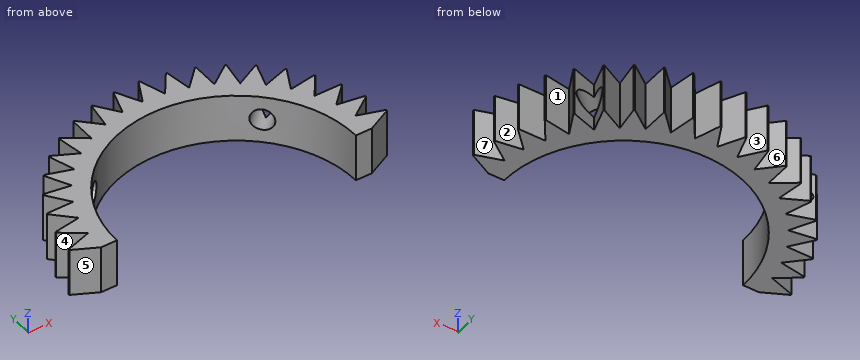
from build123d import *

# Parameters (mm, degrees)
BOSS_EXTRUDE1_DEPTH    = 7.5
CUT_EXTRUDE1_DEPTH     = 7.5
M8X1_25_TAPPED_HOLE4_D = 6.8
M8X1_25_TAPPED_HOLE5_D = 6.8


with BuildPart() as part:
    # Sketch1 → Boss-Extrude1 (new body, symmetric)
    with BuildSketch(Plane.XY):
        with BuildLine():
            Line((-50, 0), (-37.5, 0))
            ThreePointArc((-37.5, 0), (0, 37.5), (37.5, 0))
            Line((37.5, 0), (50, 0))
            ThreePointArc((50, 0), (0, 50), (-50, 0))
        make_face()
    extrude(amount=BOSS_EXTRUDE1_DEPTH, both=True)

    # Sketch2 → Cut-Extrude1 (cut, symmetric)
    with BuildSketch(Plane.XY):
        with BuildLine():
            Line((-3.75, 49.859176688), (0, 42.5))
            Line((0, 42.5), (3.75, 49.859176688))
            ThreePointArc((3.75, 49.859176688), (0, 50), (-3.75, 49.859176688))
        make_face()
        with BuildLine():
            Line((4.095862355, 49.83195673), (6.648464764, 41.976754475))
            Line((6.648464764, 41.976754475), (11.50352491, 48.658698242))
            ThreePointArc((11.50352491, 48.658698242), (7.821723252, 49.38441703), (4.095862355, 49.83195673))
        make_face()
        with BuildLine():
            Line((11.840870986, 48.577708615), (13.133222261, 40.419901943))
            Line((13.133222261, 40.419901943), (18.973794858, 46.260081157))
            ThreePointArc((18.973794858, 46.260081157), (15.450849719, 47.552825815), (11.840870986, 48.577708615))
        make_face()
        with BuildLine():
            Line((19.294318075, 46.127316094), (19.294596239, 37.867777278))
            Line((19.294596239, 37.867777278), (25.976867007, 42.722387346))
            ThreePointArc((25.976867007, 42.722387346), (22.699524987, 44.550326209), (19.294318075, 46.127316094))
        make_face()
        with BuildLine():
            Line((26.27267502, 42.541115962), (24.980873222, 34.383222261))
            Line((24.980873222, 34.383222261), (32.340302478, 38.13272657))
            ThreePointArc((32.340302478, 38.13272657), (29.389262615, 40.450849719), (26.27267502, 42.541115962))
        make_face()
        with BuildLine():
            Line((32.604111511, 37.90741237), (30.0520382, 30.0520382))
            Line((30.0520382, 30.0520382), (37.90741237, 32.604111511))
            ThreePointArc((37.90741237, 32.604111511), (35.355339059, 35.355339059), (32.604111511, 37.90741237))
        make_face()
        with BuildLine():
            Line((38.13272657, 32.340302478), (34.383222261, 24.980873222))
            Line((34.383222261, 24.980873222), (42.541115962, 26.27267502))
            ThreePointArc((42.541115962, 26.27267502), (40.450849719, 29.389262615), (38.13272657, 32.340302478))
        make_face()
        with BuildLine():
            Line((42.722387346, 25.976867007), (37.867777278, 19.294596239))
            Line((37.867777278, 19.294596239), (46.127316094, 19.294318075))
            ThreePointArc((46.127316094, 19.294318075), (44.550326209, 22.699524987), (42.722387346, 25.976867007))
        make_face()
        with BuildLine():
            Line((46.260081157, 18.973794858), (40.419901943, 13.133222261))
            Line((40.419901943, 13.133222261), (48.577708615, 11.840870986))
            ThreePointArc((48.577708615, 11.840870986), (47.552825815, 15.450849719), (46.260081157, 18.973794858))
        make_face()
        with BuildLine():
            Line((48.658698242, 11.50352491), (41.976754475, 6.648464764))
            Line((41.976754475, 6.648464764), (49.83195673, 4.095862355))
            ThreePointArc((49.83195673, 4.095862355), (49.38441703, 7.821723252), (48.658698242, 11.50352491))
        make_face()
        with BuildLine():
            Line((49.859176688, 3.75), (42.5, 0))
            Line((42.5, 0), (49.859176688, -3.75))
            ThreePointArc((49.859176688, -3.75), (50, 0), (49.859176688, 3.75))
        make_face()
        with BuildLine():
            Line((-49.859176688, -3.75), (-42.5, 0))
            Line((-42.5, 0), (-49.859176688, 3.75))
            ThreePointArc((-49.859176688, 3.75), (-50, 0), (-49.859176688, -3.75))
        make_face()
        with BuildLine():
            Line((-49.83195673, 4.095862355), (-41.976754475, 6.648464764))
            Line((-41.976754475, 6.648464764), (-48.658698242, 11.50352491))
            ThreePointArc((-48.658698242, 11.50352491), (-49.38441703, 7.821723252), (-49.83195673, 4.095862355))
        make_face()
        with BuildLine():
            Line((-48.577708615, 11.840870986), (-40.419901943, 13.133222261))
            Line((-40.419901943, 13.133222261), (-46.260081157, 18.973794858))
            ThreePointArc((-46.260081157, 18.973794858), (-47.552825815, 15.450849719), (-48.577708615, 11.840870986))
        make_face()
        with BuildLine():
            Line((-46.127316094, 19.294318075), (-37.867777278, 19.294596239))
            Line((-37.867777278, 19.294596239), (-42.722387346, 25.976867007))
            ThreePointArc((-42.722387346, 25.976867007), (-44.550326209, 22.699524987), (-46.127316094, 19.294318075))
        make_face()
        with BuildLine():
            Line((-42.541115962, 26.27267502), (-34.383222261, 24.980873222))
            Line((-34.383222261, 24.980873222), (-38.13272657, 32.340302478))
            ThreePointArc((-38.13272657, 32.340302478), (-40.450849719, 29.389262615), (-42.541115962, 26.27267502))
        make_face()
        with BuildLine():
            Line((-37.90741237, 32.604111511), (-30.0520382, 30.0520382))
            Line((-30.0520382, 30.0520382), (-32.604111511, 37.90741237))
            ThreePointArc((-32.604111511, 37.90741237), (-35.355339059, 35.355339059), (-37.90741237, 32.604111511))
        make_face()
        with BuildLine():
            Line((-32.340302478, 38.13272657), (-24.980873222, 34.383222261))
            Line((-24.980873222, 34.383222261), (-26.27267502, 42.541115962))
            ThreePointArc((-26.27267502, 42.541115962), (-29.389262615, 40.450849719), (-32.340302478, 38.13272657))
        make_face()
        with BuildLine():
            Line((-25.976867007, 42.722387346), (-19.294596239, 37.867777278))
            Line((-19.294596239, 37.867777278), (-19.294318075, 46.127316094))
            ThreePointArc((-19.294318075, 46.127316094), (-22.699524987, 44.550326209), (-25.976867007, 42.722387346))
        make_face()
        with BuildLine():
            Line((-18.973794858, 46.260081157), (-13.133222261, 40.419901943))
            Line((-13.133222261, 40.419901943), (-11.840870986, 48.577708615))
            ThreePointArc((-11.840870986, 48.577708615), (-15.450849719, 47.552825815), (-18.973794858, 46.260081157))
        make_face()
        with BuildLine():
            Line((-11.50352491, 48.658698242), (-6.648464764, 41.976754475))
            Line((-6.648464764, 41.976754475), (-4.095862355, 49.83195673))
            ThreePointArc((-4.095862355, 49.83195673), (-7.821723252, 49.38441703), (-11.50352491, 48.658698242))
        make_face()
    extrude(amount=CUT_EXTRUDE1_DEPTH, both=True, mode=Mode.SUBTRACT)

    # M8x1.25 Tapped Hole4 (through all)
    with Locations(Plane(origin=(-19.445436483, 19.445436483, 0), x_dir=(0, 0, -1), z_dir=(0.707106781, -0.707106781, 0))):
        with Locations((0, 0)):
            Hole(M8X1_25_TAPPED_HOLE4_D / 2)

    # M8x1.25 Tapped Hole5 (through all)
    with Locations(Plane(origin=(19.445436483, 19.445436483, 0), x_dir=(0, 0, -1), z_dir=(-0.707106781, -0.707106781, 0))):
        with Locations((0, 0)):
            Hole(M8X1_25_TAPPED_HOLE5_D / 2)


solid = part.part
The listing builds one solid part. Answer for the finished solid, in the listing's coordinates (mm). Face numbers are marked on the shaded views. A direction names the side the tool comes from. Round coordinates to 2 decimals unless told otherwise and drop trailing zeros. Write each loop counter-clockwise with the first axis right and the second up, starting at its lowest first coordinate (ties: lowest second). Pieces come first, ordered by that corner, then holes. Notation, with made-up numbers: M -16.5,39.5 L 25.5,39.5 A14 cw 25.5,65.5 Z; hole C 78,2 d10. An arc over 180 degrees is marked long. Write each question's results on one line, items separated by ' | '. Start each with the question number.
Item 1: Straight lines are drawn through the part: L1, parallel to X at y = 30, z = 2.5; L2, parallel to X at y = 45.5, z = -4.5; L3, parallel to X at y = 44, z = 0. For each, find the intervals that lie inside material, in ascending order. Write a range as [from, to].
Item 2: For a pull along X with two mould halves and no side action, classify the marked faces 5, 6 and 7 as pulls with the +X half, pulls with the -X half, needs draft (parallel to the pull), parting line crosses it, or undercut.
Item 3: Flat-ended cylindrical pins translate along their axes: pin 1 Ø4 at (y, z) = (27, -3) entering from +X; pin 2 Ø6 at (x, z) = (-36.5, 5.5) entering from -Y; pin 3 Ø4 at (y, z) = (41.5, -3) entering from +X; pin 4 Ø1.5 at (y, z) = (23, 0) entering from -X. Find the tip coordinate at first contact, or state that the pin passes through.
Item 4: A cutting plane is placed at A-A on y = 5. Write down the section's boundary in (x, z), and give its area (3 significant figures).
Item 5: For the marked faces 1, 2, 3 and 4, determine the directions among +Z, -Z, +X, -X, +Y, -Y from which every point of the face is accessible in a straight line to the end or side of a thin tool.
Item 6: A cutting plane is placed at B-B on x = 9.5. Write down the section's boundary in (y, z), and give its area (3 significant figures).
Item 7: A cutting plane is placed at C-C on z = -1.75. State how many separate pieces and enclosed holes the cut face has, and give its area (3 significant figures).
Check sheet entries:
1) L1: [-36.94, -33.26], [-26.74, -22.5], [22.5, 26.74], [33.26, 36.94] | L2: [-19.29, -18.21], [-12.33, -9.21], [-5.5, -1.53], [1.53, 5.5], [9.21, 12.33], [18.21, 19.29] | L3: [-19.29, -16.71], [-12.57, -8.12], [-5.99, -0.76], [0.76, 5.99], [8.12, 12.57], [16.71, 19.29]
2) face 5: pulls with the -X half | face 6: undercut | face 7: pulls with the +X half
3) pin 1: x = 42.72 | pin 2: y = 0 | pin 3: x = 26.27 | pin 4: x = -41.1
4) outline: M -47.05,-7.5 L -37.17,-7.5 L -37.17,7.5 L -47.05,7.5 Z; M 37.17,-7.5 L 47.05,-7.5 L 47.05,7.5 L 37.17,7.5 Z | area: 297 mm²
5) face 1: +Z, -Z | face 2: +Z, -Z, +X | face 3: +Z, -Z, +Y | face 4: +Z, -Z, -X
6) outline: M 36.28,-7.5 L 45.9,-7.5 L 45.9,7.5 L 36.28,7.5 Z | area: 144 mm²
7) separate pieces: 3 | enclosed holes: 0 | area: 1,060 mm²
